```python
from build123d import *

# Parameters (mm, degrees)
SKETCH_1_R      = 2.6
SKETCH_1_R_2    = 0.85
EXTRUDE_1_DEPTH = 3


with BuildPart() as part:
    # 草图1 → 凸台-拉伸1 (new body)
    with BuildSketch(Plane(origin=(0, 0, 0), x_dir=(1, 0, 0), z_dir=(0, 1, 0))):
        with BuildLine():
            Line((14.641409653, 2.5), (-14.641409653, 2.5))
            ThreePointArc((-14.641409653, 2.5), (-26.541683504, 7.620386051), (-31.005944031, 19.782016246))
            ThreePointArc((-31.005944031, 19.782016246), (-34.76320991, 23.992985156), (-38.991825792, 20.255591176))
            ThreePointArc((-38.991825792, 20.255591176), (-33.246595423, 4.255838584), (-17.646646706, -2.5))
            Line((-17.646646706, -2.5), (17.646646706, -2.5))
            ThreePointArc((17.646646706, -2.5), (33.246595423, 4.255838584), (38.991825792, 20.255591176))
            ThreePointArc((38.991825792, 20.255591176), (34.76320991, 23.992985156), (31.005944031, 19.782016246))
            ThreePointArc((31.005944031, 19.782016246), (26.541683504, 7.620386051), (14.641409653, 2.5))
        make_face()
        with Locations(Location((35, 20, 0), (0, 0, 270))):
            Circle(SKETCH_1_R, mode=Mode.SUBTRACT)
        with Locations(Location((-35, 20, 0), (0, 0, 270))):
            Circle(SKETCH_1_R, mode=Mode.SUBTRACT)
        with Locations(Location((0, 0, 0), (0, 0, 270))):
            Circle(SKETCH_1_R_2, mode=Mode.SUBTRACT)
    extrude(amount=EXTRUDE_1_DEPTH)


solid = part.part
```
Could you check a few things on this model? Use its own coordinates, in mm. A direction names the side the tool comes from. Round coordinates to 2 decimals unless told otherwise and drop trailing zeros. Write each loop counter-clockwise with the first axis right and the second up, starting at its lowest first coordinate (ties: lowest second). Pieces come first, ordered by that corner, then holes. Notation, with made-up numbers: M -18.5,27 L 13.5,27 A12 ccw 13.5,38 Z; hole C 44,-3.75 d8. An arc over 180 degrees is marked long. Answer in a Markdown table with one row per item. Add a question column.
Q1. Will these pins go through, and if not, where does the flat tip stop? pin 1 Ø0.9 at (x, y) = (-0.5, 1.5) entering from -Z; pin 2 Ø10 at (x, z) = (20, -0.5) entering from -Y; pin 3 Ø1.5 at (y, z) = (1, -3) entering from -X; pin 4 Ø1.5 at (y, z) = (1.5, -21) entering from +X.
Q2. Imagine slicing it at C-C (y = 2.15). Please give me the cut outline in (x, z), then the cut area to 3 significant figures.
Q3. If I drill on line 1 (X direction, y = 1.1, z = -20); line 2 (Z direction, x = 14, y = 2.5); line 3 (X direction, y = 2.65, z = -13), over which ranges is the centre line in solid material (lowest first)? Write a range as from..to.
Q4. Imagine slicing it at A-A (x = 0). Please give me the cut outline in (y, z), then the cut area to 3 significant figures.
Q5. If we mould it in two halves opening along Z, with no side actions, what happens to faces 3 (the cylindrical face through (35.78, 1.48, -17.52)), 4 (the cylindrical face through (-34.22, 1.48, -17.52)), 5 (the flat face through (-3, 3, -2)), 6 (the flat face through (0, 1, 2.5))? For each: +Z half, -Z half, draft (parallel to the pull), parting line (faces both ways), or undercut.
Q6. Imagine slicing it at D-D (z = 0). Please give me the cut outline in (x, y).
Q7. On a 3-axis mill with a long thin cutter (end or side, diameter ignored), from which of +Z, -Z, +X, -X, +Y, -Y can I reach the whole of each face in a straight line? I mean faces 1 (the cylindrical face through (-0.83, 1.48, -0.18)), 2 (the flat face through (0, 1, -2.5)). Say none if no direction works.
Q8. Imagine slicing it at B-B (z = -21.25). Please give me the cut outline in (x, y).
Values:
| question | item | result |
|---|---|---|
| 1 | pin 1 | z = -2.5 |
| 1 | pin 2 | y = 0 |
| 1 | pin 3 | x = -32.76 |
| 1 | pin 4 | x = 38.99 |
| 2 | outline | M -38.99,-20.26 A4 ccw -31.01,-19.78 A16.39 cw -14.64,-2.5 L 14.64,-2.5 A16.39 cw 31.01,-19.78 A4 ccw 38.99,-20.26 A21.39 ccw 17.65,2.5 L -17.65,2.5 A21.39 ccw Z; hole C -35,-20 d5.2; hole C 0,0 d1.7; hole C 35,-20 d5.2 |
| 2 | area | 595 mm^2 |
| 3 | line 1 | -39.01..-37.6, -32.4..-31, 31..32.4, 37.6..39.01 |
| 3 | line 2 | -2.5..2.5 |
| 3 | line 3 | -38.21..-29.94, 29.94..38.21 |
| 4 | outline | M 0,-2.5 L 3,-2.5 L 3,-0.85 L 0,-0.85 Z; M 0,0.85 L 3,0.85 L 3,2.5 L 0,2.5 Z |
| 4 | area | 9.90 mm^2 |
| 5 | face 3 | undercut |
| 5 | face 4 | undercut |
| 5 | face 5 | draft |
| 5 | face 6 | +Z half |
| 6 | outline | M -27.68,0 L -0.85,0 L -0.85,3 L -27.68,3 Z; M 0.85,0 L 27.68,0 L 27.68,3 L 0.85,3 Z |
| 7 | face 1 | +Y, -Y |
| 7 | face 2 | -Z, +Y, -Y |
| 8 | outline | M -38.8,0 L -37.28,0 L -37.28,3 L -38.8,3 Z; M -32.72,0 L -31.2,0 L -31.2,3 L -32.72,3 Z; M 31.2,0 L 32.72,0 L 32.72,3 L 31.2,3 Z; M 37.28,0 L 38.8,0 L 38.8,3 L 37.28,3 Z |
